Here's the drawing with two shaded views (mm, measured from the low corner). I have some questions. Round coordinates to 2 decimals unless told otherwise and drop trailing zeros. Loops run counter-clockwise (first coordinate to the right, second up) from the corner with the lowest first, then second, coordinate; pieces in that order, holes last.
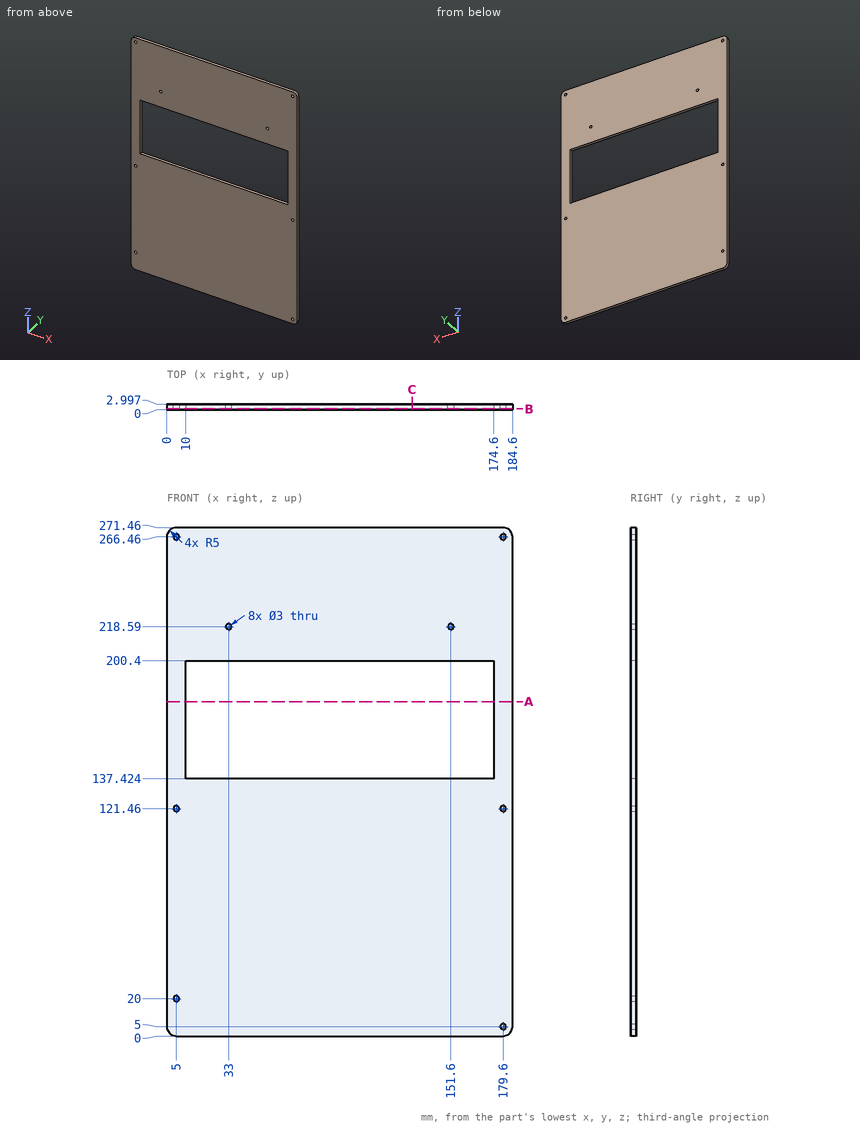
Item 1: If I drill on line 1 along Z through (x, y) = (27.5, 2.75); line 2 along X through (y, z) = (2.05, 160); line 3 along Z through (x, y) = (33, 1.65), over which ranges is the centre line in solid material (lowest first)?
Results list:
line 1: z = 0 to 137.42, 200.4 to 271.46
line 2: x = 0 to 10, 174.6 to 184.6
line 3: z = 0 to 137.42, 200.4 to 217.09, 220.09 to 271.46
Item 2: If we section it at C-C, the plane x = 131: Please give me the cut outline in (y, z).
Results list:
outline: (0, 0) - (3, 0) - (3, 137.42) - (0, 137.42) - close; (0, 200.4) - (3, 200.4) - (3, 271.46) - (0, 271.46) - close
Item 3: Will this pin go through, and if not, where does the flat tip stop? pin 1 (5 mm diameter, centred on x = 179.6, z = 5, fed in from -Y).
Results list:
pin 1: stops at y = 0
Item 4: If we section it at B-B, the plane y = 0.45: Count the separate pieces of the cut face and the enclosed holes in it, then the cut area to 3 significant figures.
Results list:
separate pieces: 1
enclosed holes: 9
area: 39,700 mm2
Item 5: If we section it at A-A, the plane z = 178.5: Please give me the cut outline in (x, y).
Results list:
outline: (0, 0) - (10, 0) - (10, 3) - (0, 3) - close; (174.6, 0) - (184.6, 0) - (184.6, 3) - (174.6, 3) - close
